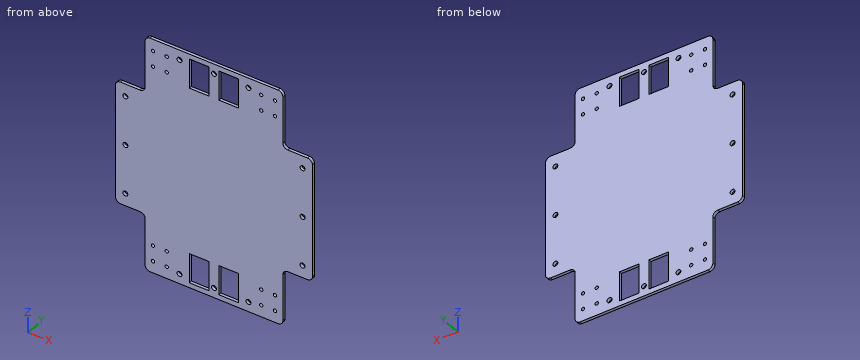
```python
from build123d import *

# Parameters (mm, degrees)
SKETCH_1_R          = 1.7
SKETCH_1_R_2        = 2.5
SKETCH_1_W          = 20
SKETCH_1_H          = 30
EXTRUDE_2_DEPTH     = 3
SKETCH_3_W          = 30
SKETCH_3_H          = 10
CUT_EXTRUDE_2_DEPTH = 3


with BuildPart() as part:
    # 草图1 → 凸台-拉伸2 (new body)
    with BuildSketch(Plane(origin=(0, 0, 0), x_dir=(1, 0, 0), z_dir=(0, 1, 0))):
        with BuildLine():
            Line((-75, 80), (-95, 80))
            ThreePointArc((-95, 80), (-98.535533906, 78.535533906), (-100, 75))
            Line((-100, 75), (-100, -75))
            ThreePointArc((-100, -75), (-98.535533906, -78.535533906), (-95, -80))
            Line((-95, -80), (-75, -80))
            ThreePointArc((-75, -80), (-71.464466094, -81.464466094), (-70, -85))
            Line((-70, -85), (-70, -115))
            ThreePointArc((-70, -115), (-68.535533906, -118.535533906), (-65, -120))
            Line((-65, -120), (65, -120))
            ThreePointArc((65, -120), (68.535533906, -118.535533906), (70, -115))
            Line((70, -115), (70, -85))
            ThreePointArc((70, -85), (71.464466094, -81.464466094), (75, -80))
            Line((75, -80), (95, -80))
            ThreePointArc((95, -80), (98.535533906, -78.535533906), (100, -75))
            Line((100, -75), (100, 75))
            ThreePointArc((100, 75), (98.535533906, 78.535533906), (95, 80))
            Line((95, 80), (75, 80))
            ThreePointArc((75, 80), (71.464466094, 81.464466094), (70, 85))
            Line((70, 85), (70, 115))
            ThreePointArc((70, 115), (68.535533906, 118.535533906), (65, 120))
            Line((65, 120), (-65, 120))
            ThreePointArc((-65, 120), (-68.535533906, 118.535533906), (-70, 115))
            Line((-70, 115), (-70, 85))
            ThreePointArc((-70, 85), (-71.464466094, 81.464466094), (-75, 80))
        make_face()
        with Locations(Location((-62, -108, 0), (0, 0, 270))):
            Circle(SKETCH_1_R, mode=Mode.SUBTRACT)
        with Locations(Location((-48, -108, 0), (0, 0, 270))):
            Circle(SKETCH_1_R, mode=Mode.SUBTRACT)
        with Locations(Location((-62, -92, 0), (0, 0, 270))):
            Circle(SKETCH_1_R, mode=Mode.SUBTRACT)
        with Locations(Location((-48, -92, 0), (0, 0, 270))):
            Circle(SKETCH_1_R, mode=Mode.SUBTRACT)
        with Locations(Location((-35, -110, 0), (0, 0, 270))):
            Circle(SKETCH_1_R_2, mode=Mode.SUBTRACT)
        with Locations((-15, -100)):
            Rectangle(SKETCH_1_W, SKETCH_1_H, mode=Mode.SUBTRACT)
        with Locations(Location((-90, -50, 0), (0, 0, 270))):
            Circle(SKETCH_1_R_2, mode=Mode.SUBTRACT)
        with Locations(Location((0, -110, 0), (0, 0, 270))):
            Circle(SKETCH_1_R_2, mode=Mode.SUBTRACT)
        with Locations((15, -100)):
            Rectangle(SKETCH_1_W, SKETCH_1_H, mode=Mode.SUBTRACT)
        with Locations(Location((35, -110, 0), (0, 0, 270))):
            Circle(SKETCH_1_R_2, mode=Mode.SUBTRACT)
        with Locations(Location((48, -108, 0), (0, 0, 270))):
            Circle(SKETCH_1_R, mode=Mode.SUBTRACT)
        with Locations(Location((62, -108, 0), (0, 0, 270))):
            Circle(SKETCH_1_R, mode=Mode.SUBTRACT)
        with Locations(Location((48, -92, 0), (0, 0, 270))):
            Circle(SKETCH_1_R, mode=Mode.SUBTRACT)
        with Locations(Location((62, -92, 0), (0, 0, 270))):
            Circle(SKETCH_1_R, mode=Mode.SUBTRACT)
        with Locations(Location((90, -50, 0), (0, 0, 270))):
            Circle(SKETCH_1_R_2, mode=Mode.SUBTRACT)
        with Locations(Location((-90, 0, 0), (0, 0, 270))):
            Circle(SKETCH_1_R_2, mode=Mode.SUBTRACT)
        with Locations(Location((-90, 50, 0), (0, 0, 270))):
            Circle(SKETCH_1_R_2, mode=Mode.SUBTRACT)
        with Locations(Location((-62, 92, 0), (0, 0, 270))):
            Circle(SKETCH_1_R, mode=Mode.SUBTRACT)
        with Locations(Location((-62, 108, 0), (0, 0, 270))):
            Circle(SKETCH_1_R, mode=Mode.SUBTRACT)
        with Locations(Location((-48, 108, 0), (0, 0, 270))):
            Circle(SKETCH_1_R, mode=Mode.SUBTRACT)
        with Locations(Location((-48, 92, 0), (0, 0, 270))):
            Circle(SKETCH_1_R, mode=Mode.SUBTRACT)
        with Locations(Location((-35, 110, 0), (0, 0, 270))):
            Circle(SKETCH_1_R_2, mode=Mode.SUBTRACT)
        Polygon((-5, 115), (-5, 100), (-5, 85), (-25, 85), (-25, 115), align=None, mode=Mode.SUBTRACT)
        with Locations(Location((90, 0, 0), (0, 0, 270))):
            Circle(SKETCH_1_R_2, mode=Mode.SUBTRACT)
        with Locations(Location((90, 50, 0), (0, 0, 270))):
            Circle(SKETCH_1_R_2, mode=Mode.SUBTRACT)
        with Locations((15, 100)):
            Rectangle(SKETCH_1_W, SKETCH_1_H, mode=Mode.SUBTRACT)
        with Locations(Location((0, 110, 0), (0, 0, 270))):
            Circle(SKETCH_1_R_2, mode=Mode.SUBTRACT)
        with Locations(Location((35, 110, 0), (0, 0, 270))):
            Circle(SKETCH_1_R_2, mode=Mode.SUBTRACT)
        with Locations(Location((48, 92, 0), (0, 0, 270))):
            Circle(SKETCH_1_R, mode=Mode.SUBTRACT)
        with Locations(Location((62, 92, 0), (0, 0, 270))):
            Circle(SKETCH_1_R, mode=Mode.SUBTRACT)
        with Locations(Location((48, 108, 0), (0, 0, 270))):
            Circle(SKETCH_1_R, mode=Mode.SUBTRACT)
        with Locations(Location((62, 108, 0), (0, 0, 270))):
            Circle(SKETCH_1_R, mode=Mode.SUBTRACT)
    extrude(amount=EXTRUDE_2_DEPTH)

    # 草图3 → 切除-拉伸2 (cut)
    with BuildSketch(Plane(origin=(0, 3, 0), x_dir=(1, 0, 0), z_dir=(0, 1, 0))):
        with Locations((85, 80)):
            Rectangle(SKETCH_3_W, SKETCH_3_H)
        with BuildLine():
            Line((95, 62.5), (100, 62.5))
            Line((100, 62.5), (100, 75))
            Line((100, 75), (70, 75))
            Line((70, 75), (70, 67.5))
            ThreePointArc((70, 67.5), (71.464466094, 63.964466094), (75, 62.5))
            Line((75, 62.5), (95, 62.5))
        make_face()
        with BuildLine():
            Line((100, 57.5), (100, 62.5))
            Line((100, 62.5), (95, 62.5))
            ThreePointArc((95, 62.5), (98.535533906, 61.035533906), (100, 57.5))
        make_face()
        with Locations((-85, 80)):
            Rectangle(SKETCH_3_W, SKETCH_3_H)
        with BuildLine():
            Line((-70, 75), (-100, 75))
            Line((-100, 75), (-100, 62.5))
            Line((-100, 62.5), (-95, 62.5))
            Line((-95, 62.5), (-75, 62.5))
            ThreePointArc((-75, 62.5), (-71.464466094, 63.964466094), (-70, 67.5))
            Line((-70, 67.5), (-70, 75))
        make_face()
        with BuildLine():
            Line((-95, 62.5), (-100, 62.5))
            Line((-100, 62.5), (-100, 57.5))
            ThreePointArc((-100, 57.5), (-98.535533906, 61.035533906), (-95, 62.5))
        make_face()
        with BuildLine():
            Line((-95, -62.5), (-100, -62.5))
            Line((-100, -62.5), (-100, -75))
            Line((-100, -75), (-70, -75))
            Line((-70, -75), (-70, -67.5))
            ThreePointArc((-70, -67.5), (-71.464466094, -63.964466094), (-75, -62.5))
            Line((-75, -62.5), (-95, -62.5))
        make_face()
        with Locations((-85, -80)):
            Rectangle(SKETCH_3_W, SKETCH_3_H)
        with BuildLine():
            Line((-100, -57.5), (-100, -62.5))
            Line((-100, -62.5), (-95, -62.5))
            ThreePointArc((-95, -62.5), (-98.535533906, -61.035533906), (-100, -57.5))
        make_face()
        with Locations((85, -80)):
            Rectangle(SKETCH_3_W, SKETCH_3_H)
        with BuildLine():
            Line((70, -75), (100, -75))
            Line((100, -75), (100, -62.5))
            Line((100, -62.5), (95, -62.5))
            Line((95, -62.5), (75, -62.5))
            ThreePointArc((75, -62.5), (71.464466094, -63.964466094), (70, -67.5))
            Line((70, -67.5), (70, -75))
        make_face()
        with BuildLine():
            Line((95, -62.5), (100, -62.5))
            Line((100, -62.5), (100, -57.5))
            ThreePointArc((100, -57.5), (98.535533906, -61.035533906), (95, -62.5))
        make_face()
    extrude(amount=-CUT_EXTRUDE_2_DEPTH, mode=Mode.SUBTRACT)


solid = part.part
```
Here's how the part is built. I have some questions about the finished solid (model axes, mm). Give positions to 0.01 mm unless a question says otherwise; leave off trailing zeros. Write each loop counter-clockwise with the first axis right and the second up, starting at its lowest first coordinate (ties: lowest second). Pieces come first, ordered by that corner, then holes.
(1) Will these pins go through, and if not, where does the flat tip stop? pin 1 (1 mm diameter, centred on y = 1, z = -71.5, fed in from -X); pin 2 (4 mm diameter, centred on x = 35, z = -110, fed in from -Y).
Output values:
pin 1: stops at x = -70
pin 2: passes through
(2) Imagine slicing it at B-B, the plane y = 1.3. Count the separate pieces of the cut face and the enclosed holes in it, and give its area (3 significant figures).
Output values:
separate pieces: 1
enclosed holes: 32
area: 38,300 mm2
(3) Imagine slicing it at C-C, the plane z = -79. Write out the boundary of the cut face in (x, y).
Output values:
outline: (-70, 0) - (70, 0) - (70, 3) - (-70, 3) - close
(4) Imagine slicing it at A-A, the plane z = 50. Write out the boundary of the cut face in (x, y), and give its area (3 significant figures).
Output values:
outline: (-100, 0) - (-92.5, 0) - (-92.5, 3) - (-100, 3) - close; (-87.5, 0) - (87.5, 0) - (87.5, 3) - (-87.5, 3) - close; (92.5, 0) - (100, 0) - (100, 3) - (92.5, 3) - close
area: 570 mm2
(5) If I drill on L1, parallel to X at y = 0.8, z = 110; L2, parallel to X at y = 0.9, z = 85.5; L3, parallel to Z at x = -12, y = 1.7, over which ranges is the centre line in solid material (lowest first)?
Output values:
L1: x = -70 to -37.5, -32.5 to -25, -5 to -2.5, 2.5 to 5, 25 to 32.5, 37.5 to 70
L2: x = -70 to -25, -5 to 5, 25 to 70
L3: z = -120 to -115, -85 to 85, 115 to 120
